Can you work these out from the model? Positions are in its coordinate system, mm. Coordinates: 2 decimals unless noted, no trailing zeros. Order: outer loops, then holes, each group sorted by start corner. A loop starts at its lowest first (then second) coordinate and runs counter-clockwise, first axis right, second up. Notation, with made-up numbers: (57.25, 13) - (66.25, 13) arc R8 cw to (66.25, 18) - close; hole circle Ø10 at (-21.5, 67). An arc over 180 degrees is marked (long way). Use a Markdown table: item, result. Add a question column.
(1) If I drill on L1, parallel to Y at x = 0, z = 157.5; L2, parallel to Y at x = -84, z = 249.5; L3, parallel to X at y = -109, z = 258, over which ranges is the centre line in solid material (lowest first)? Write a range as [from, to].
(2) For pin 1 Ø4 at (y, z) = (-30.5, 106) entering from -X; pin 2 Ø3 at (y, z) = (-191.5, 131.5) entering from -X; pin 3 Ø5 at (x, y) = (12, -193.5) entering from -Z (3 decimals); pin 4 Ø1 at (x, y) = (-115.5, 170.5) entering from -Z, each with a flat end and sliding along its axis, tell me the tip position at first contact or that it passes through.
(3) I want a section at C-C (z = 133.5). List the corners of the cut face in (x, y) for me, and give its area (3 significant figures).
(4) I want a section at A-A (y = 0). List the corners of the cut face in (x, z) for me, and give its area (3 significant figures).
(5) We'd pull the mould along Y, two halves only. Please class faces 1 (the flat face through (-114, 171, 0)), 2 (the cylindrical face through (-221.722, -170.011, 175.666)), 3 (the cylindrical face through (169.59, 53.41, 179.93)): pulls with the +Y half, pulls with the -Y half, needs draft (parallel to the pull), parting line crosses it, or undercut.
```python
from build123d import *

# Parameters (mm, degrees)
SKETCH2_R           = 279.4
BOSS_EXTRUDE1_DEPTH = 355.6
SKETCH3_R           = 177.8
CUT_EXTRUDE1_DEPTH  = 532.582618226
FILLET3_R           = 25.4
FILLET4_R           = 25.4


with BuildPart() as part:
    # Sketch2 → Boss-Extrude1 (new body)
    with BuildSketch(Plane.XY):
        Circle(SKETCH2_R)
    extrude(amount=BOSS_EXTRUDE1_DEPTH)

    # Sketch3 → Cut-Extrude1 (cut, through all)
    with BuildSketch(Plane.XY.offset(355.6)):
        Circle(SKETCH3_R)
    extrude(amount=-CUT_EXTRUDE1_DEPTH, mode=Mode.SUBTRACT)

    # Fillet3
    fillet3_edges = [part.edges().sort_by_distance(p)[0] for p in [
        (-279.4, 0, 0),
        (-279.4, 0, 355.6),
    ]]
    fillet(fillet3_edges, radius=FILLET3_R)

    # Fillet4
    fillet4_edges = [part.edges().sort_by_distance(p)[0] for p in [
        (-177.8, 0, 0),
        (-177.8, 0, 355.6),
    ]]
    fillet(fillet4_edges, radius=FILLET4_R)


solid = part.part
```
Answers follow:
| question | item | result |
|---|---|---|
| 1 | L1 | y = [-279.4, -177.8], [177.8, 279.4] |
| 1 | L2 | y = [-266.47, -156.71], [156.71, 266.47] |
| 1 | L3 | x = [-257.26, -140.47], [140.47, 257.26] |
| 2 | pin 1 | stops at x = -277.94 |
| 2 | pin 2 | stops at x = -204.85 |
| 2 | pin 3 | stops at z = 0.935 |
| 2 | pin 4 | stops at z = 0 |
| 3 | outline | circle Ø558.8 at (0, 0); hole circle Ø355.6 at (0, 0) |
| 3 | area | 146,000 mm² |
| 4 | outline | (-279.4, 25.4) arc R25.4 ccw to (-254, 0) - (-203.2, 0) arc R25.4 ccw to (-177.8, 25.4) - (-177.8, 330.2) arc R25.4 ccw to (-203.2, 355.6) - (-254, 355.6) arc R25.4 ccw to (-279.4, 330.2) - close; (177.8, 25.4) arc R25.4 ccw to (203.2, 0) - (254, 0) arc R25.4 ccw to (279.4, 25.4) - (279.4, 330.2) arc R25.4 ccw to (254, 355.6) - (203.2, 355.6) arc R25.4 ccw to (177.8, 330.2) - close |
| 4 | area | 71,200 mm² |
| 5 | face 1 | needs draft |
| 5 | face 2 | parting line crosses it |
| 5 | face 3 | undercut |
